Verification items for the finished model (mm, model axes). Face numbers are marked on the shaded views. A direction names the side the tool comes from. Round coordinates to 2 decimals unless told otherwise and drop trailing zeros.
Autodesk Inventor part; units mm, degrees
ref_plane "YZ Plane" through (0, 0, 0) normal (1, 0, 0) x (0, 1, 0)
ref_plane "XZ Plane" through (0, 0, 0) normal (0, 1, 0) x (-1, 0, 0)
ref_plane "XY Plane" through (0, 0, 0) normal (0, 0, 1) x (1, 0, 0)
sketch "Skizze1" plane through (0, 0, 0) normal (0, 0, 1) x (1, 0, 0)
  arc A0 (0, 180) -> (-180, 0) centre (0, 0) ccw
  line L0 (-260.7351, 0) -> (43.4558, 0)
  line L1 (0, -43.4558) -> (0, 260.7351)
  dimension "d0" = 180
  dimension "d1" = 90
sketch "Skizze2" plane through (0, 0, 0) normal (0, 1, 0) x (-1, 0, 0)
  line L0 (0, -42) -> (0, 42)
  circle A0 centre (180, 0) radius 7
  line L1 (252, 0) -> (-42, 0)
  circle A1 centre (180, 0) radius 12
  line L2 (191.9553, 0) -> (168, 0)
  line L3 (173, 0) -> (160, 0)
  line L4 (173, 2) -> (173, 0)
  line L5 (187, 0) -> (200, 0)
  line L6 (187, 2) -> (187, 0)
  circle A2 centre (180, 0) radius 30
  line L7 (187, 2) -> (209.9333, 2)
  line L8 (173, 2) -> (150.0667, 2)
  point P0 (0, 0)
  point P1 (173, 0)
  point P2 (168, 0)
  point P3 (192, 0)
  point P4 (191.8322, 2)
  point P5 (168.1678, 2)
  point P6 (150, 0)
  point P7 (210, 0)
  dimension "d5" = 24
  dimension "d3" = 180
  dimension "d4" = 14
  dimension "d16" = 60
  dimension "d17" = 2
  dimension "d18" = 23
  dimension "d19" = 7
sweep "Sweeping1" add profiles "Skizze2" path "Skizze1" path curves A0 contours L6 L7 A1 L1 | A0 L4 L8 A1 L7 L6 | L1 A1 L8 L4 | L1 A2 L8 A1 | A1 L7 A2 L1
sketch "Skizze7" plane through (-168.1678, 0, 2) normal (0, 0, 1) x (1, 0, 0)
  line L0 (18.1678, 0) -> (18.1678, -3)
  line L1 (0, 0) -> (18.1011, 0)
  line L2 (168.1678, 150) -> (171.1678, 150)
  line L3 (168.1678, 168.1678) -> (168.1678, 150.0667)
  line L4 (168.1678, 210) -> (171.1678, 210)
  arc A0 (168.1678, 150.0667) -> (18.1011, 0) centre (168.1678, 0) ccw
  circle A1 centre (168.1678, 0) radius 168
  line L5 (-41.8322, 0) -> (-41.8322, -3)
  point P0 (10.1678, 15)
  point P1 (56.0828, 112.085)
  point P2 (153.1678, 158)
  dimension "d36" = 8
  dimension "d37" = 15
  dimension "d38" = 8
  dimension "d39" = 15
  dimension "d41" = 97.915
  dimension "d42" = 97.915
hole "Bohrung1" at (-158, 15, 2) at (-112.085, 112.085, 2) at (-15, 158, 2) direction (0, 0, -1) diameter 4 depth 8
sketch "Skizze8" plane through (-209.9333, 0, 2) normal (0, 0, 1) x (1, 0, 0)
  line L0 (-0.0667, 0) -> (-0.0667, -3)
  line L1 (0, 0) -> (18.1011, 0)
  line L2 (209.9333, 209.9333) -> (209.9333, 191.8322)
  line L3 (209.9333, 210) -> (212.9333, 210)
  arc A0 (209.9333, 168.1678) -> (41.7654, 0) centre (209.9333, 0) ccw
  circle A1 centre (209.9333, 0) radius 200.8827
  point P0 (209.9333, 0)
  point P1 (9.6113, 15)
  point P2 (67.8861, 142.044)
  point P3 (194.9333, 200.3219)
  dimension "d51" = 15
  dimension "d52" = 15
  dimension "d54" = 142.044
  dimension "d59" = 401.7655
  dimension "d60" = 142.0471
hole "Bohrung3" at (-200.3219, 15, 2) at (-142.0471, 142.044, 2) at (-15, 200.3219, 2) direction (0, 0, -1) diameter 4 depth 8
properties part number "ph-l_mk1"
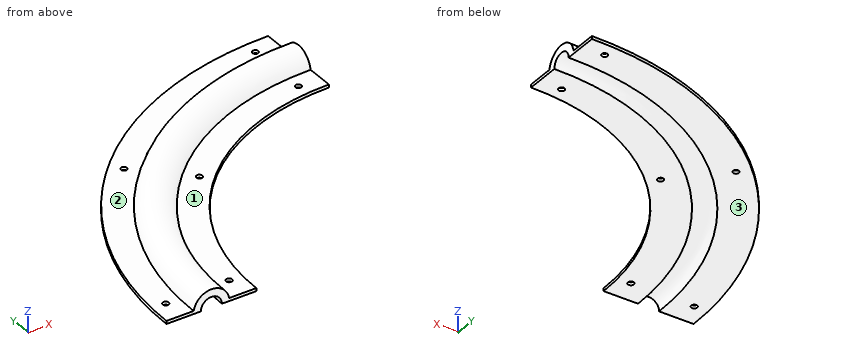
Q1. Tool access check on the marked faces 1, 2 and 3. Record the directions out of +Z, -Z, +X, -X, +Y, -Y that give a thin tool (end or side, any length) a straight path to the whole face; none if there is none.
Recorded:
face 1: +Z, +X, -Y
face 2: +Z, -X, +Y
face 3: -Z, +X, -X, +Y, -Y
Q2. Material ranges on line 1 along X through (y, z) = (15, 1.25); line 2 along Z through (x, y) = (-143, 47); line 3 along X through (y, z) = (15, 0.75), recorded low to high.
Recorded:
line 1: x = -209.44 to -202.32, -198.32 to -186.28, -172.46 to -160, -156 to -149.27
line 2: z = 0 to 2
line 3: x = -209.45 to -202.32, -198.32 to -186.36, -172.39 to -160, -156 to -149.26
Q3. Depth check by flat-ended pin: P1, Ø4, axis at y = 126.5, z = 5.5, coming from the +X side; P2, Ø1.5, axis at y = 102, z = 1, coming from the +X side; P3, Ø2, axis at x = -72.5, z = 7.5, coming from the +Y side. Enter the tip coordinate at first touch or a pass-through.
Recorded:
P1: stops at x = -109.89
P2: stops at x = -109.3
P3: stops at y = 175.83
